from build123d import *

# Parameters (mm, degrees)
F0_R     = 11.049
F1_DEPTH = 1.5748
F2_R     = 5.3975
F3_DEPTH = 1.27
F4_R     = 4.064
F4_R_2   = 2.8575
F5_DEPTH = 2.54


with BuildPart() as f1:
    # F0 (on Top) → F1 (new body)
    with BuildSketch(Plane.XY):
        Circle(F0_R)
    extrude(amount=F1_DEPTH)

    # F2 (on face) → F3 (join)
    with BuildSketch(Plane.XY.offset(1.5748)):
        Circle(F2_R)
    extrude(amount=F3_DEPTH)

    # F4 (on face) → F5 (join)
    with BuildSketch(Plane.XY.offset(2.8448)):
        Circle(F4_R)
        Circle(F4_R_2, mode=Mode.SUBTRACT)
    extrude(amount=F5_DEPTH)


solid = f1.part
The listing builds one solid part. Answer for the finished solid, in the listing's coordinates (mm). A direction names the side the tool comes from. Round coordinates to 2 decimals unless told otherwise and drop trailing zeros. Order: outer loops, then holes, each group sorted by start corner. A loop starts at its lowest first (then second) coordinate and runs counter-clockwise, first axis right, second up. Notation, with made-up numbers: (-9.5, 11.5) -> (2.5, 11.5) arc R21 ccw to (2.5, 38.5) -> close; hole circle Ø6 at (-6, -14.5). An arc over 180 degrees is marked (long way). Put each result on its own line as item: value.
Q1. Determine the mould class of faces 3 (the flat face through (-2, 4, 2.845)), 4 (the cylindrical face through (-3.978, 3.648, 2.201)), 5 (the cylindrical face through (2.726, 0.858, 4.097)) for opening direction X: pulls with the +X half, pulls with the -X half, needs draft (parallel to the pull), parting line crosses it, or undercut.
Results list:
face 3: needs draft
face 4: parting line crosses it
face 5: undercut
Q2. Each of these flat-tipped pins is pushed along its axis until it touches: P1, Ø2, axis at x = -2.5, z = 1.5, coming from the -Y side; P2, Ø2, axis at x = 5.5, y = 8, coming from the +Z side. Where does it stop, or does it pass through?
Results list:
P1: y = -10.95
P2: z = 1.57
Q3. Section D-D, the plane z = 0.7 is taken. Write down the section's boundary in (x, y).
Results list:
outline: circle Ø22.1 at (0, 0)
Q4. Section A-A, the plane x = 0 is taken. Write down the section's boundary in (y, z).
Results list:
outline: (-11.05, 0) -> (11.05, 0) -> (11.05, 1.57) -> (5.4, 1.57) -> (5.4, 2.84) -> (4.06, 2.84) -> (4.06, 5.38) -> (2.86, 5.38) -> (2.86, 2.84) -> (-2.86, 2.84) -> (-2.86, 5.38) -> (-4.06, 5.38) -> (-4.06, 2.84) -> (-5.4, 2.84) -> (-5.4, 1.57) -> (-11.05, 1.57) -> close
Q5. Which of the six approach directions +Z, -Z, +X, -X, +Y, -Y give full straight-line access (tool end or side, diameter ignored) to faces 1 (the flat face through (0, 0, 2.845)), 2 (the flat face through (0, 0, 0))?
Results list:
face 1: +Z
face 2: -Z, +X, -X, +Y, -Y
Q6. Consider line 1 along Y through (x, z) = (0, 3.55); line 2 along Z through (x, y) = (-5.25, -4.5); line 3 along X through (y, z) = (2.5, 3.05). Determine where each line is inside the solid, lowest interval first.
Results list:
line 1: -4.06 to -2.86, 2.86 to 4.06
line 2: 0 to 1.57
line 3: -3.2 to -1.38, 1.38 to 3.2
Q7. Section C-C, the plane z = 3.8 is taken. Write down the section's boundary in (x, y) (1 decimal), and give its area (3 significant figures).
Results list:
outline: circle Ø8.1 at (0, 0); hole circle Ø5.7 at (0, 0)
area: 26.2 mm^2
